Geometry check sheet. Reference: the model listing, model coordinates, mm. A direction names the side the tool comes from. Round coordinates to 2 decimals unless told otherwise and drop trailing zeros. Loops run counter-clockwise (first coordinate to the right, second up) from the corner with the lowest first, then second, coordinate; pieces in that order, holes last. Notation, with made-up numbers: M 62.25,59.5 L 107.25,59.5 A22 ccw 107.25,92.5 Z; hole C -17.75,75 d4. An arc over 180 degrees is marked long. Use one line per item in the form item = value. Start each with the question number.
1. Material ranges on line 1 (Y direction, x = -11.5, z = -3); line 2 (X direction, y = -0.75, z = 2.25); line 3 (X direction, y = -1.25, z = -3.25), recorded low to high.
2. Cross-section at C-C (z = -0.75). Record the boundary of the cut face in (x, y), then the cut area to 3 significant figures.
3. Set-up check for faces 1 (the cylindrical face through (10.113, 7.452, -3.284)), 2 (the cylindrical face through (15.397, 0.186, 1.397)), 3 (the cylindrical face through (-15.397, 0.186, 1.397)): record each of +Z, -Z, +X, -X, +Y, -Y from which the full face is reachable in a straight line by a thin tool's end or side.
4. Cross-section at A-A (y = -2.5). Record the boundary of the cut face in (x, z).
5. Cross-section at B-B (x = 15). Record the boundary of the cut face in (y, z), then the cut area to 3 significant figures.
6. Go/stop test with flat-tipped pins: pin 1 (1.6 mm diameter, centred on x = 10.93, y = -7.11, fed in from -Z); pin 2 (2 mm diameter, centred on y = 1.397, z = 1.016, fed in from +X). Record where each tip stops, or that it passes through.
7. Cross-section at D-D (z = -2.75). State how many separate pieces and enclosed holes the cut face has, then the cut area to 3 significant figures.
8. Draft check along X on faces 4 (the conical face through (-11.048, -7.216, -1.591)), 5 (the flat face through (0, 0, 4.572)), 6 (the flat face through (16.65, 0, 0)). Enter one of: pulls with the +X half, pulls with the -X half, needs draft (parallel to the pull), parting line crosses it, or undercut.
```python
from build123d import *

# Parameters (mm, degrees)
F0_W     = 33.2994
F0_H     = 19.304
F1_DEPTH = 4.572
F2_R     = 1.27
F3_DEPTH = 2.54
F5_D     = 1.778
F5_DEPTH = 2.54
F5_TIP   = 0.5341650903
F8_R     = 1.27
F9_DEPTH = 9.145


# Not quite as in the source:
# - a pattern or mirror of a feature is missing from the dataset's text; its kind, count and spacing are read off the source's solid


with BuildPart() as f1:
    # F0 (on Top) → F1 (new body, symmetric)
    with BuildSketch(Plane.XY):
        Rectangle(F0_W, F0_H)
    extrude(amount=F1_DEPTH, both=True)

    # F2 (on face) → F3 (cut)
    with BuildSketch(Plane(origin=(-16.6497, 0, 0), x_dir=(0, -1, 0), z_dir=(-1, 0, 0))):
        with Locations((-1.397, 1.016)):
            Circle(F2_R)
    f3 = extrude(amount=-F3_DEPTH, mode=Mode.SUBTRACT)

    # F3_copies: F3 across plane
    add(f3.mirror(Plane(origin=(0, 0, 0), x_dir=(0, 0, 1), z_dir=(1, 0, 0))), mode=Mode.SUBTRACT)

    # F5
    with Locations(Plane(origin=(0, 0, -4.572), x_dir=(1, 0, 0), z_dir=(0, 0, -1))):
        with Locations((10.9347, -7.112), (10.9347, 7.112), (-10.9347, -7.112), (-10.9347, 7.112)):
            Hole(F5_D / 2, depth=F5_DEPTH)
            with Locations((0, 0, -(F5_DEPTH + F5_TIP / 2))):  # 118° drill point
                Cone(0, F5_D / 2, F5_TIP, mode=Mode.SUBTRACT)

    # F8 (on face) → F9 (cut, through all)
    with BuildSketch(Plane(origin=(0, 0, -4.572), x_dir=(1, 0, 0), z_dir=(0, 0, -1))):
        with Locations((-14.732, 1.778)):
            Circle(F8_R)
        with Locations((-14.732, -4.572)):
            Circle(F8_R)
        with Locations((14.732, 1.778)):
            Circle(F8_R)
        with Locations((14.732, -4.572)):
            Circle(F8_R)
    extrude(amount=-F9_DEPTH, mode=Mode.SUBTRACT)


solid = f1.part
```
Reported:
q1.line_1 = -9.65 to -7.8, -6.43 to 6.43, 7.8 to 9.65
q1.line_2 = -16.65 to -15.48, -13.99 to 13.99, 15.48 to 16.65
q1.line_3 = -16.65 to -15.89, -13.58 to 13.58, 15.89 to 16.65
q2.outline = M -16.65,-9.65 L 16.65,-9.65 L 16.65,9.65 L -16.65,9.65 Z; hole C -14.73,-1.78 d2.54; hole C -14.73,4.57 d2.54; hole C 14.73,-1.78 d2.54; hole C 14.73,4.57 d2.54
q2.area = 623 mm²
q3.face_1 = -Z
q3.face_2 = +X
q3.face_3 = -X
q4.outline = M -16.65,-4.57 L -15.78,-4.57 L -15.78,4.57 L -16.65,4.57 Z; M -13.69,-4.57 L 13.69,-4.57 L 13.69,4.57 L -13.69,4.57 Z; M 15.78,-4.57 L 16.65,-4.57 L 16.65,4.57 L 15.78,4.57 Z
q5.outline = M -9.65,-4.57 L -3.02,-4.57 L -3.02,4.57 L -9.65,4.57 Z; M -0.54,-4.57 L 3.33,-4.57 L 3.33,4.57 L -0.54,4.57 Z; M 5.81,-4.57 L 9.65,-4.57 L 9.65,4.57 L 5.81,4.57 Z; hole C 1.4,1.02 d2.54
q5.area = 126 mm²
q6.pin_1 = -1.98
q6.pin_2 = 14.11
q7.separate_pieces = 1
q7.enclosed_holes = 8
q7.area = 613 mm²
q8.face_4 = undercut
q8.face_5 = needs draft
q8.face_6 = pulls with the +X half
